from build123d import *

# Parameters (mm, degrees)
F0_R     = 63.5
F0_R_2   = 6.35
F1_DEPTH = 6.35
F2_R     = 6.34999
F4_DEPTH = 12.7


# Not quite as in the source:
# - a fillet or chamfer is up to 0.001 mm smaller than in the source, because OpenCascade refuses the exact size


with BuildPart() as f1:
    # F0 (on Front) → F1 (new body, symmetric)
    with BuildSketch(Plane.XZ):
        Circle(F0_R)
        Circle(F0_R_2, mode=Mode.SUBTRACT)
    extrude(amount=F1_DEPTH, both=True)

    # F2 (radius 6.35 in the source; OpenCascade refuses exactly that, so slightly less here)
    f2_edges = [f1.edges().sort_by_distance(p)[0] for p in [
        (-63.5, -6.35, 0),
        (-63.5, 6.35, 0),
    ]]
    fillet(f2_edges, radius=F2_R)

    # F3 (on Right) → F4 (join, symmetric)
    with BuildSketch(Plane.YZ):
        Polygon((-12.7, -12.7), (0, -12.7), (12.7, -12.7), (12.7, 88.9), (-12.7, 88.9), align=None)
    extrude(amount=F4_DEPTH, both=True)


solid = f1.part
For this review, take the finished solid that the model builds, in its own axes (mm). A direction names the side the tool comes from. Give positions to 0.01 mm unless a question says otherwise; leave off trailing zeros. Loops run counter-clockwise (first coordinate to the right, second up) from the corner with the lowest first, then second, coordinate; pieces in that order, holes last.
Item 1: Insertion check: pin 1 (2 mm diameter, centred on y = 1.5, z = 38.5, fed in from +X); pin 2 (7 mm diameter, centred on x = 4.5, y = 10, fed in from -Z); pin 3 (3 mm diameter, centred on x = 20, z = 46.5, fed in from +Y). Each pin has a flat end and moves straight along its axis. Give the tip position at first contact, or say it passes through.
Item 2: Tool access review of faces 1 (the flat face through (12.7, 8, 50)), 2 (the flat face through (0, -12.7, 39)), 3 (the flat face through (0, 9, -12.7)), 4 (the flat face through (0, -10, -12.7)), 5 (the flat face through (-12.7, 8, 50)): name each direction out of +Z, -Z, +X, -X, +Y, -Y from which nothing blocks a thin tool from reaching the whole face with its end or side.
Item 3: For line 1 along Y through (x, z) = (-5.5, -46); line 2 along Z through (x, y) = (0.5, 7), list the stretches that pass through material, from the lowest coordinate up.
Item 4: Take a section at C-C, the plane y = -10.25. State the section outline as (x, z) points.
Calculated:
1. pin 1: stops at x = 51.07
1. pin 2: stops at z = -12.7
1. pin 3: stops at y = 6.35
2. face 1: +Z, +X, +Y
2. face 2: +Z, -Z, +X, -X, -Y
2. face 3: -Z, +X, -X, +Y
2. face 4: -Z, +X, -X, -Y
2. face 5: +Z, -X, +Y
3. line 1: y = -6.35 to 6.35
3. line 2: z = -12.7 to 88.9
4. outline: (-12.7, -12.7) - (12.7, -12.7) - (12.7, 88.9) - (-12.7, 88.9) - close
